from build123d import *

# Parameters (mm, degrees)
BOSS_EXTRUDE1_DEPTH = 50.8
SKETCH2_W           = 12.7
SKETCH2_H           = 6.35
BOSS_EXTRUDE2_DEPTH = 6.35
SKETCH3_R           = 1.499997
CUT_EXTRUDE1_DEPTH  = 71.299547696
FILLET1_R           = 2.54


with BuildPart() as part:
    # Sketch1 → Boss-Extrude1 (new body)
    with BuildSketch(Plane(origin=(0, 0, 0), x_dir=(0, 0, -1), z_dir=(1, 0, 0))):
        Polygon((0, 0), (-42.8625, 0), (-42.8625, 4.7625), (-4.7625, 4.7625), (-4.7625, 30.1625), (0, 30.1625), align=None)
    extrude(amount=BOSS_EXTRUDE1_DEPTH)

    # Sketch2 → Boss-Extrude2 (add)
    with BuildSketch(Plane(origin=(0, 4.7625, 0), x_dir=(1, 0, 0), z_dir=(0, 1, 0))):
        with Locations((25.4, -20.6375)):
            Rectangle(SKETCH2_W, SKETCH2_H)
    extrude(amount=BOSS_EXTRUDE2_DEPTH)

    # Sketch3 → Cut-Extrude1 (cut, through all)
    with BuildSketch(Plane.XY.offset(4.7625)):
        with Locations((25.4, 23.8125)):
            Circle(SKETCH3_R)
    extrude(amount=-CUT_EXTRUDE1_DEPTH, mode=Mode.SUBTRACT)

    # Fillet1
    fillet1_edges = [part.edges().sort_by_distance(p)[0] for p in [
        (19.05, 11.1125, 20.6375),
        (25.4, 11.1125, 23.8125),
        (31.75, 11.1125, 20.6375),
        (25.4, 11.1125, 17.4625),
    ]]
    fillet(fillet1_edges, radius=FILLET1_R)


solid = part.part
Can you work these out from the model? Positions are in its coordinate system, mm. A direction names the side the tool comes from. Round coordinates to 2 decimals unless told otherwise and drop trailing zeros. Write each loop counter-clockwise with the first axis right and the second up, starting at its lowest first coordinate (ties: lowest second). Pieces come first, ordered by that corner, then holes. Notation, with made-up numbers: (89.5, -12) -> (111.5, -12) arc R5 ccw to (111.5, -8) -> close; hole circle Ø3 at (24.5, -7.5). An arc over 180 degrees is marked (long way). Use one line per item in the form item = value. Start each with the question number.
Q1. Imagine slicing it at C-C (z = 25.5). Please give me the cut outline in (x, y).
Q2. Imagine slicing it at B-B (x = 12). Please give me the cut outline in (y, z), then the cut area to 3 significant figures.
Q3. Which directions (+Z, -Z, +X, -X, +Y, -Y) give clear straight access to the entire face, cutting with the end or side of a thin tool? Please do faces 1 (the face through (25, 11.112, 21)), 2 (the face through (31.75, 7, 21)), 3 (the face through (25.49, 10.35, 18.19)), 4 (the face through (19.05, 7, 21)).
Q4. I'm going to push flat-ended pins straight in: P1, Ø1.1, axis at y = 6.5, z = 19.5, coming from the -X side; P2, Ø7.5, axis at x = 21.5, y = 14.5, coming from the +Z side; P3, Ø19, axis at x = 13, z = 19.5, coming from the +Y side. Where does each tip first touch, or does it pass through?
Q5. We'd pull the mould along X, two halves only. Please class faces 5 (the face through (31.307, 10.006, 20.593)), 6 (the face through (25, 15, 0)), 7 (the face through (25.2, 25.3, 2.4)), 8 (the face through (19.493, 10.006, 20.593)): +X half, -X half, draft (parallel to the pull), parting line (faces both ways), or undercut.
Q6. Imagine slicing it at A-A (x = 25.4). Please give me the cut outline in (y, z), then the cut area to 3 significant figures.
Q7. If I drill on probe 1 along Y at (x, z) = (25.4, 2.1); probe 2 along Z at (x, y) = (22, 20.5), over which ranges is the centre line in solid material (lowest first)? Write a range as [from, to].
Worked out:
q1.outline = (0, 0) -> (50.8, 0) -> (50.8, 4.76) -> (0, 4.76) -> close
q2.outline = (0, 0) -> (30.16, 0) -> (30.16, 4.76) -> (4.76, 4.76) -> (4.76, 42.86) -> (0, 42.86) -> close
q2.area = 325 mm^2
q3.face_1 = +Z, +X, -X, +Y
q3.face_2 = +Z, +X, +Y
q3.face_3 = +X, -X, +Y
q3.face_4 = +Z, -X, +Y
q4.P1 = 19.05
q4.P2 = 22.58
q4.P3 = 11.11
q5.face_5 = +X half
q5.face_6 = draft
q5.face_7 = undercut
q5.face_8 = -X half
q6.outline = (0, 0) -> (22.31, 0) -> (22.31, 4.76) -> (4.76, 4.76) -> (4.76, 17.46) -> (8.57, 17.46) arc R2.54 ccw to (11.11, 20) -> (11.11, 21.27) arc R2.54 ccw to (8.57, 23.81) -> (4.76, 23.81) -> (4.76, 42.86) -> (0, 42.86) -> close; (25.31, 0) -> (30.16, 0) -> (30.16, 4.76) -> (25.31, 4.76) -> close
q6.area = 348 mm^2
q7.probe_1 = [0, 22.31], [25.31, 30.16]
q7.probe_2 = [0, 4.76]
